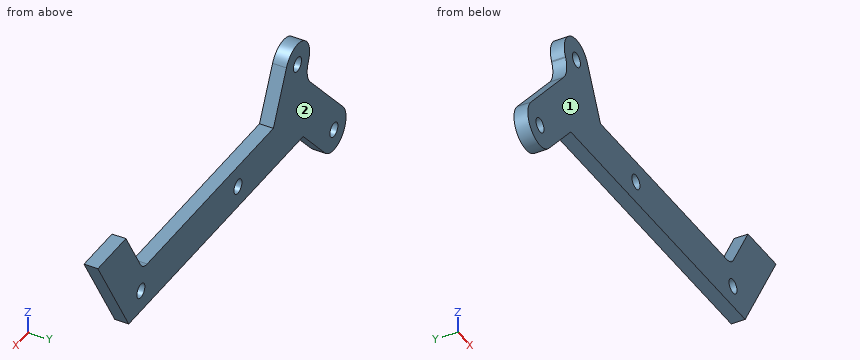
from build123d import *

# Parameters (mm, degrees)
BOSS_EXTRUDE1_DEPTH   = 1.5875
M4X0_7_TAPPED_HOLE1_D = 3.3
M4X0_7_TAPPED_HOLE2_D = 3.3


with BuildPart() as part:
    # Sketch1 → Boss-Extrude1 (new body, symmetric)
    with BuildSketch(Plane(origin=(0, 0, 0), x_dir=(1, 0, 0), z_dir=(0, 1, 0))):
        with BuildLine():
            Line((0, 0), (-11.547005384, 0))
            Line((-11.547005384, 0), (-17.558665062, 10.4125))
            ThreePointArc((-17.558665062, 10.4125), (-18.720795719, 11.574630657), (-20.308295719, 12))
            Line((-20.308295719, 12), (-72.308295719, 12))
            Line((-72.308295719, 12), (-77.698457708, 0.440760311))
            ThreePointArc((-77.698457708, 0.440760311), (-84.343088233, -1.977687418), (-86.761535579, 4.666942928))
            Line((-86.761535579, 4.666942928), (-86.675516364, 4.851411729))
            ThreePointArc((-86.675516364, 4.851411729), (-86.262765717, 7.708815155), (-87.498464442, 10.318061424))
            Line((-87.498464442, 10.318061424), (-100.938587731, 25.181055478))
            ThreePointArc((-100.938587731, 25.181055478), (-100.583555179, 32.243204718), (-93.521405939, 31.888172166))
            Line((-93.521405939, 31.888172166), (-84.579852673, 22))
            Line((-84.579852673, 22), (-12.701705922, 22))
            Line((-12.701705922, 22), (0, 0))
        make_face()
    extrude(amount=BOSS_EXTRUDE1_DEPTH, both=True)

    # M4x0.7 Tapped Hole1 (through all)
    with Locations(Plane(origin=(0, 1.5875, 0), x_dir=(1, 0, 0), z_dir=(0, 1, 0))):
        with Locations((-17.701705922, 17), (-57.701705922, 17)):
            Hole(M4X0_7_TAPPED_HOLE1_D / 2)

    # M4x0.7 Tapped Hole2 (through all)
    with Locations(Plane(origin=(0, 1.5875, 0), x_dir=(1, 0, 0), z_dir=(0, 1, 0))):
        with Locations((-82.229996835, 2.553851709), (-97.229996835, 28.534613822)):
            Hole(M4X0_7_TAPPED_HOLE2_D / 2)


solid = part.part
Geometry: final body of the model. Coordinates: model frame, mm. Face numbers are marked on the shaded views. Coordinates: 2 decimals unless noted, no trailing zeros. Loops run counter-clockwise (first coordinate to the right, second up) from the corner with the lowest first, then second, coordinate; pieces in that order, holes last. Notation, with made-up numbers: M 44.5,62 L 103.5,62 A23 ccw 103.5,97 Z; hole C -35.75,72 d4. An arc over 180 degrees is marked long. One line per item, written item: value. Start each with the question number.
1) Pin query (flat end, axial travel): P1, Ø4.5, axis at x = -57.7, z = -17, coming from the -Y side. Return the tip coordinate at first contact, or that it passes through.
2) Material intervals for L1, parallel to X at y = 1.4, z = -17; L2, parallel to Z at x = -53, y = 0.95; L3, parallel to Z at x = -57, y = 1.05, sorted ascending. Write a range as from..to.
3) Cut plane D-D (x = -44). Return loops of the section in (y, z), then the cut area to 4 significant figures.
4) Draft query along Y for the marked faces 1 and 2. Return one class per face: released by +Y, released by -Y, zero draft, split by the parting line, or undercut.
5) Cut plane C-C (z = -17). Return loops of the section in (x, y).
6) Cut plane A-A (z = -7.5). Return loops of the section in (x, y).
7) Cut plane B-B (y = 0.3). Count the separate pieces of the cut face and the enclosed holes in it, then the cut area to 3 significant figures.
Evaluation:
1. P1: y = -1.59
2. L1: -93.54..-59.35, -56.05..-19.35, -16.05..-9.81
2. L2: -22..-12
2. L3: -22..-18.49, -15.51..-12
3. outline: M -1.59,-22 L 1.59,-22 L 1.59,-12 L -1.59,-12 Z
3. area: 31.75 mm^2
4. face 1: released by -Y
4. face 2: released by +Y
5. outline: M -93.54,-1.59 L -59.35,-1.59 L -59.35,1.59 L -93.54,1.59 Z; M -56.05,-1.59 L -19.35,-1.59 L -19.35,1.59 L -56.05,1.59 Z; M -16.05,-1.59 L -9.81,-1.59 L -9.81,1.59 L -16.05,1.59 Z
6. outline: M -86.24,-1.59 L -74.41,-1.59 L -74.41,1.59 L -86.24,1.59 Z; M -15.88,-1.59 L -4.33,-1.59 L -4.33,1.59 L -15.88,1.59 Z
7. separate pieces: 1
7. enclosed holes: 4
7. area: 1,230 mm^2
